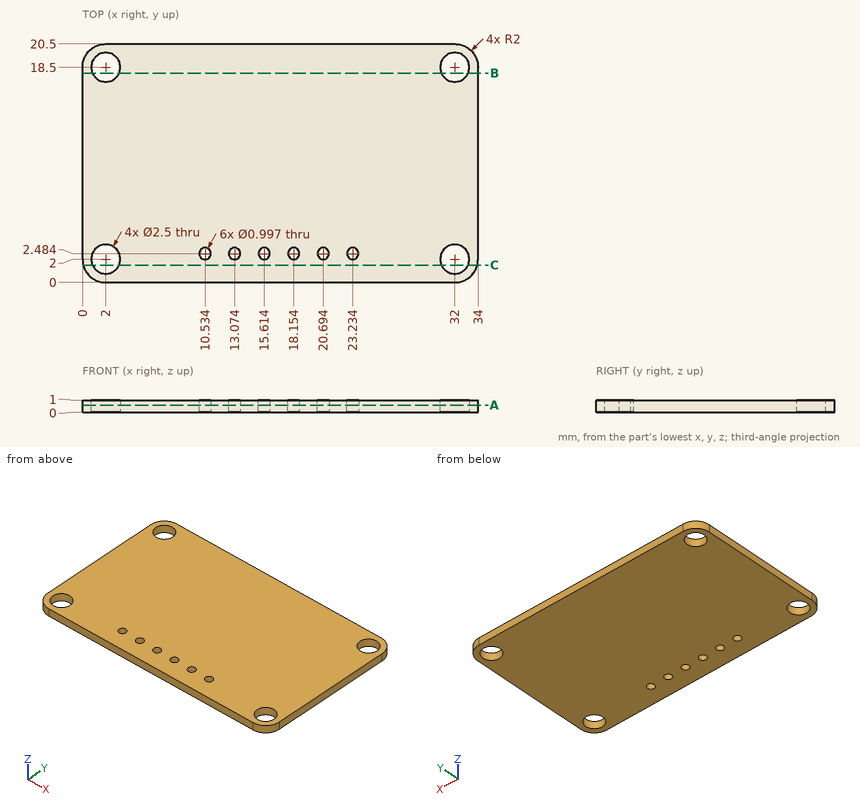
Drawing for the job (mm, zero at the part's lowest x, y, z). Coordinates: 2 decimals unless noted, no trailing zeros. Write each loop counter-clockwise with the first axis right and the second up, starting at its lowest first coordinate (ties: lowest second). Pieces come first, ordered by that corner, then holes. Notation, with made-up numbers: (10.5, 79) -> (24.5, 79) arc R16 cw to (24.5, 87) -> close; hole circle Ø6 at (76.5, 70). An arc over 180 degrees is marked (long way). One line per item, written item: value. Start each with the question number.
1) Flat gauge pin, fed straight in: pin 1 Ø1.5 at (x, y) = (2, 18.5) entering from +Z. Where does the tip first touch, or does it go through?
2) Slice it at B-B on y = 18. Write the cut outline in (x, z) (1 decimal).
3) Slice it at C-C on y = 1.5. Write the cut outline in (x, z) (1 decimal).
4) Probe probe 1 along Y at (x, z) = (2, 0.5); probe 2 along X at (y, z) = (18.25, 0.95) (1 decimal); probe 3 along X at (y, z) = (18, 0.75) (1 decimal). List the from-to ranges inside material, lowest first.
5) Slice it at A-A on z = 0.6. Count the separate pieces of the cut face and the enclosed holes in it, then the cut area to 3 significant figures.
Answers follow:
1. pin 1: through
2. outline: (0, 0) -> (0.9, 0) -> (0.9, 1) -> (0, 1) -> close; (3.1, 0) -> (30.9, 0) -> (30.9, 1) -> (3.1, 1) -> close; (33.1, 0) -> (34, 0) -> (34, 1) -> (33.1, 1) -> close
3. outline: (0.1, 0) -> (0.9, 0) -> (0.9, 1) -> (0.1, 1) -> close; (3.1, 0) -> (30.9, 0) -> (30.9, 1) -> (3.1, 1) -> close; (33.1, 0) -> (33.9, 0) -> (33.9, 1) -> (33.1, 1) -> close
4. probe 1: 0 to 0.75, 3.25 to 17.25, 19.75 to 20.5
4. probe 2: 0 to 0.8, 3.2 to 30.8, 33.2 to 34
4. probe 3: 0 to 0.9, 3.1 to 30.9, 33.1 to 34
5. separate pieces: 1
5. enclosed holes: 10
5. area: 669 mm2
